CAD build for the part. Positions are in the model's coordinates, mm. Coordinates: 2 decimals unless noted, no trailing zeros. Order: outer loops, then holes, each group sorted by start corner. A loop starts at its lowest first (then second) coordinate and runs counter-clockwise, first axis right, second up. Notation, with made-up numbers: (33.25, 74) - (63.25, 74) arc R37 cw to (63.25, 113) - close; hole circle Ø9 at (31.25, 0). An arc over 180 degrees is marked (long way). Write each question's results on one line, items separated by ' | '. Start each with the question number.
Q1. Band-saw the part on C-C, the plane x = -0.75. Write the cut outline in (y, z), then the cut area to 3 significant figures.
Q2. Pin check, flat tip, straight feed: P1, Ø4.5, axis at x = -1, z = -1, coming from the -Y side. Stop position of the tip, or through.
Q3. Band-saw the part on D-D, the plane y = -0.45. Write the cut outline in (x, z).
Q4. Wall check: probe 1 along Y at (x, z) = (-0.75, 5.25); probe 2 along Z at (x, y) = (-6.25, 1.9); probe 3 along Z at (x, y) = (-4.25, 1.15). Give the ranges that are in metal, low to high.
Q5. Band-saw the part on A-A, the plane y = 0.85. Write the cut outline in (x, z) (3 decimals), then the cut area to 4 significant figures.
Q6. Band-saw the part on B-B, the plane z = 1.5. Write the cut outline in (x, y) (3 decimals), then the cut area to 3 significant figures.
```python
from build123d import *

# Parameters (mm, degrees)
SKETCH1_W           = 14.75
SKETCH1_H           = 14.5
BOSS_EXTRUDE1_DEPTH = 2
CUT_EXTRUDE1_DEPTH  = 2
SKETCH3_W           = 11
SKETCH3_H           = 0.7
CUT_EXTRUDE2_DEPTH  = 12
SKETCH4_R           = 0.4
BOSS_EXTRUDE2_DEPTH = 0.65


with BuildPart() as part:
    # Sketch1 → Boss-Extrude1 (new body)
    with BuildSketch(Plane(origin=(0, 0, 0), x_dir=(1, 0, 0), z_dir=(0, 1, 0))):
        Rectangle(SKETCH1_W, SKETCH1_H)
    extrude(amount=BOSS_EXTRUDE1_DEPTH)

    # Sketch2 → Cut-Extrude1 (cut)
    with BuildSketch(Plane(origin=(0, 2, 0), x_dir=(1, 0, 0), z_dir=(0, 1, 0))):
        Polygon((-7.375, -6.25), (2.375, -6.25), (3.375, -7.25), (-7.375, -7.25), align=None)
    extrude(amount=-CUT_EXTRUDE1_DEPTH, mode=Mode.SUBTRACT)

    # Sketch3 → Cut-Extrude2 (cut)
    with BuildSketch(Plane.XY.offset(7.25)):
        with Locations((-0.95, 1)):
            Rectangle(SKETCH3_W, SKETCH3_H)
    extrude(amount=-CUT_EXTRUDE2_DEPTH, mode=Mode.SUBTRACT)

    # Sketch4 → Boss-Extrude2 (add)
    with BuildSketch(Plane.XZ):
        with Locations((-4.95, 3.25)):
            Circle(SKETCH4_R)
        with Locations((3.05, 3.25)):
            Circle(SKETCH4_R)
    extrude(amount=BOSS_EXTRUDE2_DEPTH)


solid = part.part
```
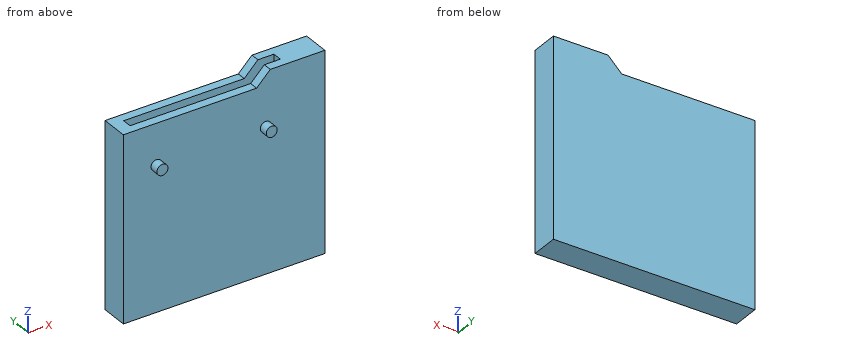
Results below:
1) outline: (0, -7.25) - (2, -7.25) - (2, 6.25) - (1.35, 6.25) - (1.35, -4.75) - (0.65, -4.75) - (0.65, 6.25) - (0, 6.25) - close | area: 19.3 mm²
2) P1: stops at y = 0
3) outline: circle Ø0.8 at (-4.95, 3.25); circle Ø0.8 at (3.05, 3.25)
4) probe 1: y = 0 to 0.65, 1.35 to 2 | probe 2: z = -7.25 to 6.25 | probe 3: z = -7.25 to -4.75
5) outline: (-7.375, -7.25) - (7.375, -7.25) - (7.375, 7.25) - (4.55, 7.25) - (4.55, -4.75) - (-6.45, -4.75) - (-6.45, 6.25) - (-7.375, 6.25) - close | area: 80.95 mm²
6) outline: (-7.375, 0) - (7.375, 0) - (7.375, 2) - (-7.375, 2) - close; hole (-6.45, 0.65) - (4.55, 0.65) - (4.55, 1.35) - (-6.45, 1.35) - close | area: 21.8 mm²
